Check sheet for the modelled part. Datum: model origin and axes. Units: mm. A direction names the side the tool comes from. Coordinates: 2 decimals unless noted, no trailing zeros. Write each loop counter-clockwise with the first axis right and the second up, starting at its lowest first coordinate (ties: lowest second). Pieces come first, ordered by that corner, then holes. Notation, with made-up numbers: M 57.25,-22 L 93.25,-22 A29 cw 93.25,6 Z; hole C 78,49.25 d8. An arc over 180 degrees is marked long. Answer as CSV lines item,"result". Start each with the question number.
Q1. Sectioned sample at A-A, the plane z = 9.5. Record the cut outline in (x, y).
Q2. Depth check by flat-ended pin: pin 1 Ø2 at (x, z) = (7.5, 39.5) entering from +Y; pin 2 Ø2 at (y, z) = (-14, 73) entering from -X; pin 3 Ø9 at (x, y) = (13.5, 6) entering from +Z. Enter the tip coordinate at first touch or a pass-through.
Q3. Access from +Z, -Z, +X, -X, +Y, -Y to the whole of each face (thin tool, end or side, straight path). Record for faces 5 (the flat face through (4, 10.207, -1)), 6 (the flat face through (4, 6, 61.5)), 7 (the flat face through (-53, -1.793, 36)).
Q4. Mould release check, pull along Z, two halves, no side actions. Record for faces 1 (the flat face through (57, -13, 0)), 2 (the flat face through (4, 2.207, 70)), 3 (the flat face through (4, 2.207, 45)), 4 (the flat face through (4, -23.793, 35)): pulls with the +Z half, pulls with the -Z half, needs draft (parallel to the pull), parting line crosses it, or undercut.
Q5. Thickness scan on line 1 along X through (y, z) = (-17.5, 44.5); line 2 along Y through (x, z) = (-40, 63); line 3 along Z through (x, y) = (-34, -17.5). Record the ranges inside material, lowest first. Write a range as from..to.
from build123d import *

# Parameters (mm, degrees)
EXTRUDE_1_DEPTH     = 73
SKETCH_2_W          = 118
SKETCH_2_H          = 34
EXTRUDE_2_DEPTH     = 3
SKETCH_3_W          = 4
SKETCH_3_H          = 8
SKETCH_3_W_2        = 1.701544984
CUT_EXTRUDE_1_DEPTH = 122
SKETCH_4_W          = 24
SKETCH_4_H          = 11
EXTRUDE_3_DEPTH     = 10
CUT_EXTRUDE_2_DEPTH = 72
CUT_EXTRUDE_3_DEPTH = 5
CHAMFER_1_SIZE      = 2


with BuildPart() as part:
    # Эскиз1 → Бобышка-Вытянуть1 (new body)
    with BuildSketch(Plane.XY):
        Polygon((-49.206262386, -23.793189369), (54.793737614, -23.793189369), (54.793737614, -1.793189369), (61.793737614, -1.793189369), (61.793737614, 10.206810631), (-56.206262386, 10.206810631), (-56.206262386, -1.793189369), (-49.206262386, -1.793189369), align=None)
    extrude(amount=EXTRUDE_1_DEPTH)

    # Эскиз2 → Бобышка-Вытянуть2 (add)
    with BuildSketch(Plane(origin=(0, 0, 0), x_dir=(-1, 0, 0), z_dir=(0, 0, -1))):
        with Locations((-2.793737614, -6.793189369)):
            Rectangle(SKETCH_2_W, SKETCH_2_H)
    extrude(amount=EXTRUDE_2_DEPTH)

    # Эскиз3 → Вырез-Вытянуть1 (cut)
    with BuildSketch(Plane(origin=(61.793737614, 0, 0), x_dir=(0, 0, -1), z_dir=(1, 0, 0))):
        with Locations((-69.5, 6.206810631)):
            Rectangle(SKETCH_3_W, SKETCH_3_H)
        with Locations((-64.5, 6.206810631)):
            Rectangle(SKETCH_3_W, SKETCH_3_H)
        with Locations((-59.5, 6.206810631)):
            Rectangle(SKETCH_3_W, SKETCH_3_H)
        with Locations((-54.5, 6.206810631)):
            Rectangle(SKETCH_3_W, SKETCH_3_H)
        with Locations((-49.5, 6.206810631)):
            Rectangle(SKETCH_3_W, SKETCH_3_H)
        with Locations((-44.5, 6.206810631)):
            Rectangle(SKETCH_3_W, SKETCH_3_H)
        with Locations((-39.5, 6.206810631)):
            Rectangle(SKETCH_3_W, SKETCH_3_H)
        with Locations((-34.5, 6.206810631)):
            Rectangle(SKETCH_3_W, SKETCH_3_H)
        with Locations((-29.5, 6.206810631)):
            Rectangle(SKETCH_3_W, SKETCH_3_H)
        with Locations((-24.5, 6.206810631)):
            Rectangle(SKETCH_3_W, SKETCH_3_H)
        with Locations((-19.5, 6.206810631)):
            Rectangle(SKETCH_3_W, SKETCH_3_H)
        with Locations((-14.5, 6.206810631)):
            Rectangle(SKETCH_3_W, SKETCH_3_H)
        with Locations((-9.5, 6.206810631)):
            Rectangle(SKETCH_3_W, SKETCH_3_H)
        with Locations((-4.5, 6.206810631)):
            Rectangle(SKETCH_3_W, SKETCH_3_H)
        with Locations((-0.850772492, 6.206810631)):
            Rectangle(SKETCH_3_W_2, SKETCH_3_H)
    extrude(amount=-CUT_EXTRUDE_1_DEPTH, mode=Mode.SUBTRACT)

    # Эскиз4 → Бобышка-Вытянуть3 (add)
    with BuildSketch(Plane.XY.offset(73)):
        with Locations((35.793737614, -10.293189369)):
            Rectangle(SKETCH_4_W, SKETCH_4_H)
        with Locations((-10.206262386, -10.293189369)):
            Rectangle(SKETCH_4_W, SKETCH_4_H)
    extrude(amount=EXTRUDE_3_DEPTH)

    # Эскиз5 → Вырез-Вытянуть2 (cut)
    with BuildSketch(Plane.ZY.offset(22.206262386)):
        Polygon((83, -4.793189369), (83, -9.681423082), (81.084531501, -15.793189369), (84.818796285, -15.793189369), (84.818796285, -4.793189369), align=None)
    extrude(amount=-CUT_EXTRUDE_2_DEPTH, mode=Mode.SUBTRACT)

    # Эскиз6 → Вырез-Вытянуть3 (cut)
    with BuildSketch(Plane(origin=(0, 0, -3), x_dir=(-1, 0, 0), z_dir=(0, 0, -1))):
        with BuildLine():
            Line((-59.293737614, -11.024578472), (-61.793737614, -11.024578472))
            Line((-61.793737614, -11.024578472), (-61.793737614, -14.561800266))
            Line((-61.793737614, -14.561800266), (-59.293737614, -14.561800266))
            ThreePointArc((-59.293737614, -14.561800266), (-57.525126717, -12.793189369), (-59.293737614, -11.024578472))
        make_face()
        with BuildLine():
            Line((53.706262386, -10.764633874), (56.206262386, -10.764633874))
            Line((56.206262386, -10.764633874), (56.206262386, -14.821744863))
            Line((56.206262386, -14.821744863), (53.706262386, -14.821744863))
            ThreePointArc((53.706262386, -14.821744863), (51.677706891, -12.793189369), (53.706262386, -10.764633874))
        make_face()
    extrude(amount=-CUT_EXTRUDE_3_DEPTH, mode=Mode.SUBTRACT)

    # Фаска1
    chamfer_1_edges = [part.edges().sort_by_distance(p)[0] for p in [
        (54.793737614, -23.793189369, 36.5),
        (2.793737614, -23.793189369, 73),
        (-49.206262386, -23.793189369, 36.5),
    ]]
    chamfer(chamfer_1_edges, length=CHAMFER_1_SIZE)


solid = part.part
Output:
1,outline,"M -56.21,-1.79 L -49.21,-1.79 L -49.21,-21.79 L -47.21,-23.79 L 52.79,-23.79 L 54.79,-21.79 L 54.79,-1.79 L 61.79,-1.79 L 61.79,2.21 L -56.21,2.21 Z"
2,pin 1,"stops at y = 2.21"
2,pin 2,"stops at x = -49.21"
2,pin 3,"stops at z = 73"
3,face 5,"+Z, -Z, +X, -X, +Y"
3,face 6,"+X, -X, +Y"
3,face 7,"+Z, -X, -Y"
4,face 1,"pulls with the +Z half"
4,face 2,"undercut"
4,face 3,"undercut"
4,face 4,"needs draft"
5,line 1,"x = -49.21..54.79"
5,line 2,"y = -23.79..2.21"
5,line 3,"z = -3..73"
